Read the model definition and answer for the solid it produces. Units are mm, in the model's axes. A direction names the side the tool comes from. Give positions to 0.01 mm unless a question says otherwise; leave off trailing zeros. Order: outer loops, then holes, each group sorted by start corner. A loop starts at its lowest first (then second) coordinate and runs counter-clockwise, first axis right, second up.
Item 1: Given pin 1 Ø3.5 at (y, z) = (71.5, 2.5) entering from +X; pin 2 Ø3 at (x, z) = (-2, 2) entering from -Y; pin 3 Ø3 at (x, z) = (-69, 4) entering from +Y, each flat-ended and moving along its own axis, determine where each tip first touches the part or whether it passes through.
Item 2: Which of the six approach directions +Z, -Z, +X, -X, +Y, -Y give full straight-line access (tool end or side, diameter ignored) to faces 1 (the face through (-33.036, 57.137, 3.042)), 2 (the face through (53, -17, 6)), 3 (the face through (-64, 20, 3))?
Item 3: A cutting plane is placed at C-C (y = -39). Write down the section's boundary in (x, z), plus the area to 3 significant figures.
Item 4: A cutting plane is placed at A-A (x = 0). Write down the section's boundary in (y, z).
Item 5: Find the intervals of material crossed by line 1 along Y through (x, z) = (0, 1.75); line 2 along Y through (x, z) = (-65, 3.8); line 3 along X through (y, z) = (0, 2.8), in increasing order.
Item 6: The mould has two halves that part along X. Classify faces 4 (the face through (79.935, 3.235, 2.958)), 5 (the face through (-65, -20, 3)), 6 (the face through (-60.57, 35.09, 2.96)): +X half, -X half, draft (parallel to the pull), parting line (faces both ways), or undercut.
Item 7: A cutting plane is placed at D-D (x = -41). Write down the section's boundary in (y, z), plus the area to 3 significant figures.
Item 8: A cutting plane is placed at B-B (y = 0). Write down the section's boundary in (x, z), plus the area to 3 significant figures.
Autodesk Inventor part; units mm, degrees
ref_plane "YZ Plane" through (0, 0, 0) normal (1, 0, 0) x (0, 1, 0)
ref_plane "XZ Plane" through (0, 0, 0) normal (0, 1, 0) x (-1, 0, 0)
ref_plane "XY Plane" through (0, 0, 0) normal (0, 0, 1) x (1, 0, 0)
sketch "Sketch1" plane through (0, 0, 0) normal (0, 0, 1) x (1, 0, 0)
  circle A0 centre (0, 0) radius 80
  circle A1 centre (0, 0) radius 55
  line L0 (-7.5, 73) -> (7.5, 73)
  line L1 (7.5, 73) -> (7.5, 70)
  line L2 (7.5, 70) -> (-7.5, 70)
  line L3 (-7.5, 70) -> (-7.5, 73)
  line L4 (-66.9699, 30.0048) -> (-59.4699, 42.9952)
  line L5 (-59.4699, 42.9952) -> (-56.8718, 41.4952)
  line L6 (-56.8718, 41.4952) -> (-64.3718, 28.5048)
  line L7 (-64.3718, 28.5048) -> (-66.9699, 30.0048)
  line L8 (-59.4699, -42.9952) -> (-66.9699, -30.0048)
  line L9 (-66.9699, -30.0048) -> (-64.3718, -28.5048)
  line L10 (-64.3718, -28.5048) -> (-56.8718, -41.4952)
  line L11 (-56.8718, -41.4952) -> (-59.4699, -42.9952)
  line L12 (7.5, -73) -> (-7.5, -73)
  line L13 (-7.5, -73) -> (-7.5, -70)
  line L14 (-7.5, -70) -> (7.5, -70)
  line L15 (7.5, -70) -> (7.5, -73)
  line L16 (66.9699, -30.0048) -> (59.4699, -42.9952)
  line L17 (59.4699, -42.9952) -> (56.8718, -41.4952)
  line L18 (56.8718, -41.4952) -> (64.3718, -28.5048)
  line L19 (64.3718, -28.5048) -> (66.9699, -30.0048)
  line L20 (59.4699, 42.9952) -> (66.9699, 30.0048)
  line L21 (66.9699, 30.0048) -> (64.3718, 28.5048)
  line L22 (64.3718, 28.5048) -> (56.8718, 41.4952)
  line L23 (56.8718, 41.4952) -> (59.4699, 42.9952)
  line L24 (-58.1708, 43.7452) -> (-43.1708, 43.7452)
  line L25 (-43.1708, 43.7452) -> (-43.1708, 40.7452)
  line L26 (-43.1708, 40.7452) -> (-58.1708, 40.7452)
  line L27 (-58.1708, 40.7452) -> (-58.1708, 43.7452)
  line L28 (-58.1708, -40.7452) -> (-43.1708, -40.7452)
  line L29 (-43.1708, -40.7452) -> (-43.1708, -43.7452)
  line L30 (-43.1708, -43.7452) -> (-58.1708, -43.7452)
  line L31 (-58.1708, -43.7452) -> (-58.1708, -40.7452)
  line L32 (0, 20) -> (-100, 20)
  line L33 (-100, 20) -> (-100, -20)
  line L34 (-100, -20) -> (0, -20)
  line L35 (0, -20) -> (0, 20)
  point P0 (0, 73)
  point P1 (7.5, 71.5)
  point P2 (0, 70)
  point P3 (-63.2199, 36.5)
  point P4 (-58.1708, 42.2452)
  point P5 (-60.6218, 35)
  point P6 (-63.2199, -36.5)
  point P7 (-65.6708, -29.2548)
  point P8 (-60.6218, -35)
  point P9 (0, -73)
  point P10 (-7.5, -71.5)
  point P11 (0, -70)
  point P12 (63.2199, -36.5)
  point P13 (58.1708, -42.2452)
  point P14 (60.6218, -35)
  point P15 (63.2199, 36.5)
  point P16 (65.6708, 29.2548)
  point P17 (60.6218, 35)
  point P18 (-58.1708, 42.2452)
  point P19 (-58.1708, -42.2452)
  point P20 (-51.2348, -20)
  point P21 (-77.4597, -20)
  point P22 (-77.4597, 20)
  point P23 (-51.2348, 20)
  dimension "d0" = 160
  dimension "d1" = 110
  dimension "d2" = 15
  dimension "d3" = 3
  dimension "d11" = 70
  dimension "d14" = 360
  dimension "d18" = 15
  dimension "d19" = 3
  dimension "d20" = 15
  dimension "d21" = 3
  dimension "d22" = 40
  dimension "d23" = 100
extrude "Extrusion2" add sketch "Sketch1" along normal blind 6 contours A0 L34 A1 L32 | L27 L24 L25 L26 L6 L5 | L11 L10 L28 L29 L30 L31 picked at (16.7927, -65.9701)
sketch "草圖4" plane through (0, 0, 6) normal (0, 0, 1) x (1, 0, 0)
  line L0 (63, 3) -> (66, 3)
  line L1 (66, 3) -> (66, -3)
  line L2 (66, -3) -> (63, -3)
  line L3 (63, -3) -> (63, 3)
  line L4 (28.9019, 56.0596) -> (30.4019, 58.6577)
  line L5 (30.4019, 58.6577) -> (35.5981, 55.6577)
  line L6 (35.5981, 55.6577) -> (34.0981, 53.0596)
  line L7 (34.0981, 53.0596) -> (28.9019, 56.0596)
  line L8 (-34.0981, 53.0596) -> (-35.5981, 55.6577)
  line L9 (-35.5981, 55.6577) -> (-30.4019, 58.6577)
  line L10 (-30.4019, 58.6577) -> (-28.9019, 56.0596)
  line L11 (-28.9019, 56.0596) -> (-34.0981, 53.0596)
  line L12 (-63, -3) -> (-66, -3)
  line L13 (-66, -3) -> (-66, 3)
  line L14 (-66, 3) -> (-63, 3)
  line L15 (-63, 3) -> (-63, -3)
  line L16 (-28.9019, -56.0596) -> (-30.4019, -58.6577)
  line L17 (-30.4019, -58.6577) -> (-35.5981, -55.6577)
  line L18 (-35.5981, -55.6577) -> (-34.0981, -53.0596)
  line L19 (-34.0981, -53.0596) -> (-28.9019, -56.0596)
  line L20 (34.0981, -53.0596) -> (35.5981, -55.6577)
  line L21 (35.5981, -55.6577) -> (30.4019, -58.6577)
  line L22 (30.4019, -58.6577) -> (28.9019, -56.0596)
  line L23 (28.9019, -56.0596) -> (34.0981, -53.0596)
  point P0 (0, 0)
  point P1 (63, 0)
  point P2 (31.5, 54.5596)
  point P3 (-31.5, 54.5596)
  point P4 (-63, 0)
  point P5 (-31.5, -54.5596)
  point P6 (31.5, -54.5596)
  dimension "d44" = 3
  dimension "d45" = 6
  dimension "d46" = 63
  dimension "d49" = 360
extrude "擠出6" cut sketch "草圖4" against normal blind 10 contours L0 L1 L2 L3 | L4 L5 L6 L7 | L8 L9 L10 L11 | L16 L17 L18 L19 | L20 L21 L22 L23
properties part number "back_cir_hold"
Response values:
1. pin 1: stops at x = 39.18
1. pin 2: stops at y = -80
1. pin 3: stops at y = 42.94
2. face 1: +Z, -Z
2. face 2: +Z, +X, -X, +Y, -Y
2. face 3: +Z, -Z, -X
3. outline: (-69.85, 0) - (-61.78, 0) - (-61.78, 6) - (-69.85, 6) - close; (-58.31, 0) - (-38.78, 0) - (-38.78, 6) - (-58.31, 6) - close; (38.78, 0) - (58.31, 0) - (58.31, 6) - (38.78, 6) - close; (61.78, 0) - (69.85, 0) - (69.85, 6) - (61.78, 6) - close
3. area: 331 mm2
4. outline: (-80, 0) - (-73, 0) - (-73, 6) - (-80, 6) - close; (-70, 0) - (-55, 0) - (-55, 6) - (-70, 6) - close; (55, 0) - (70, 0) - (70, 6) - (55, 6) - close; (73, 0) - (80, 0) - (80, 6) - (73, 6) - close
5. line 1: y = -80 to -73, -70 to -55, 55 to 70, 73 to 80
5. line 2: y = -46.64 to -33.42, -28.87 to -20, 20 to 28.87, 33.42 to 46.64
5. line 3: x = 55 to 63, 66 to 80
6. face 4: parting line
6. face 5: draft
6. face 6: undercut
7. outline: (-68.69, 0) - (-36.66, 0) - (-36.66, 6) - (-68.69, 6) - close; (36.66, 0) - (68.69, 0) - (68.69, 6) - (36.66, 6) - close
7. area: 384 mm2
8. outline: (55, 0) - (63, 0) - (63, 6) - (55, 6) - close; (66, 0) - (80, 0) - (80, 6) - (66, 6) - close
8. area: 132 mm2
